from build123d import *

# Parameters (mm, degrees)
F0_W     = 32
F0_H     = 25
F1_DEPTH = 390
F2_R     = 4
F3_DEPTH = 93
F4_R     = 6.5
F5_DEPTH = 40.8
F6_R     = 9
F7_DEPTH = 13
F8_R     = 6
F9_DEPTH = 76.1


with BuildPart() as f1:
    # F0 (on Right) → F1 (new body)
    with BuildSketch(Plane.YZ):
        Rectangle(F0_W, F0_H)
    extrude(amount=F1_DEPTH)

    # F2 (on face) → F3 (cut)
    with BuildSketch(Plane(origin=(0, 16, 0), x_dir=(-1, 0, 0), z_dir=(0, 1, 0))):
        with Locations((-320, 5)):
            Circle(F2_R)
        with Locations((-70, 5)):
            Circle(F2_R)
    extrude(amount=-F3_DEPTH, mode=Mode.SUBTRACT)

    # F4 (on face) → F5 (cut)
    with BuildSketch(Plane(origin=(0, 0, -12.5), x_dir=(1, 0, 0), z_dir=(0, 0, -1))):
        with Locations((20, 0)):
            Circle(F4_R)
        with Locations((370, 0)):
            Circle(F4_R)
    extrude(amount=-F5_DEPTH, mode=Mode.SUBTRACT)

    # F6 (on face) → F7 (cut)
    with BuildSketch(Plane.XY.offset(12.5)):
        with Locations((20, 0)):
            Circle(F6_R)
        with Locations((370, 0)):
            Circle(F6_R)
    extrude(amount=-F7_DEPTH, mode=Mode.SUBTRACT)

    # F8 (on face) → F9 (cut)
    with BuildSketch(Plane(origin=(0, 0, -12.5), x_dir=(1, 0, 0), z_dir=(0, 0, -1))):
        with Locations((50, 0)):
            Circle(F8_R)
        with Locations((340, 0)):
            Circle(F8_R)
    extrude(amount=-F9_DEPTH, mode=Mode.SUBTRACT)


solid = f1.part
Verification items for the finished model (mm, model axes). A direction names the side the tool comes from. Coordinates: 2 decimals unless noted, no trailing zeros. Loops run counter-clockwise (first coordinate to the right, second up) from the corner with the lowest first, then second, coordinate; pieces in that order, holes last. Notation, with made-up numbers: (-28, -19.75) -> (14, -19.75) arc R29 cw to (14, 4.25) -> close; hole circle Ø3 at (44.5, 21). An arc over 180 degrees is marked (long way). Answer as a JSON object with one key per item and string values. Group by question number.
Item 1: Sectioned sample at B-B on z = 5. Record the boundary of the cut face in (x, y).
Item 2: Sectioned sample at C-C on x = 50. Record the boundary of the cut face in (y, z).
Item 3: Sectioned sample at A-A on y = 0. State how many separate pieces and enclosed holes the cut face has, plus the area to 3 significant figures.
Item 4: Tool access check on faces 4 (the cylindrical face through (28.584, 2.703, 6.091)), 5 (the flat face through (192, 0, -12.5)). Record the directions out of +Z, -Z, +X, -X, +Y, -Y that give a thin tool (end or side, any length) a straight path to the whole face; none if there is none.
Item 5: Mould release check, pull along Y, two halves, no side actions. Record for faces 1 (the cylindrical face through (324, 0, 5)), 2 (the flat face through (192, 16, 0)), 3 (the cylindrical face through (378.314, -3.447, 6.091)): +Y half, -Y half, draft (parallel to the pull), parting line (faces both ways), or undercut.
Item 6: Depth check by flat-ended pin: pin 1 (8 mm diameter, centred on x = 20, y = 0, fed in from +Z); pin 2 (16 mm diameter, centred on x = 370, y = 0, fed in from +Z). Enter the tip coordinate at first touch or a pass-through.
Item 7: Scan lines: probe 1 along X at (y, z) = (10.5, 4.25); probe 2 along Y at (x, z) = (370, 6); probe 3 along Y at (x, z) = (20.5, -9.5). Record each from-to range of solid material in increasing order.
Evaluation:
{
 "1": {"outline": "(0, -16) -> (66, -16) -> (66, 16) -> (0, 16) -> close; (74, -16) -> (316, -16) -> (316, 16) -> (74, 16) -> close; (324, -16) -> (390, -16) -> (390, 16) -> (324, 16) -> close; hole circle Ø18 at (20, 0); hole circle Ø12 at (50, 0); hole circle Ø12 at (340, 0); hole circle Ø18 at (370, 0)"},
 "2": {"outline": "(-16, -12.5) -> (-6, -12.5) -> (-6, 12.5) -> (-16, 12.5) -> close; (6, -12.5) -> (16, -12.5) -> (16, 12.5) -> (6, 12.5) -> close"},
 "3": {"separate pieces": "5", "enclosed holes": "2", "area": "8,270 mm²"},
 "4": {"face 4": "+Z", "face 5": "-Z, +X, -X, +Y, -Y"},
 "5": {"face 1": "draft", "face 2": "+Y half", "face 3": "undercut"},
 "6": {"pin 1": "passes through", "pin 2": "stops at z = -0.5"},
 "7": {"probe 1": "x = 0 to 66.07, 73.93 to 316.07, 323.93 to 390", "probe 2": "y = -16 to -9, 9 to 16", "probe 3": "y = -16 to -6.48, 6.48 to 16"}
}
